Verification items for the finished model (mm, model axes). Face numbers are marked on the shaded views. A direction names the side the tool comes from. Round coordinates to 2 decimals unless told otherwise and drop trailing zeros. Write each loop counter-clockwise with the first axis right and the second up, starting at its lowest first coordinate (ties: lowest second). Pieces come first, ordered by that corner, then holes. Notation, with made-up numbers: (-13, 16) - (13, 16) arc R18 cw to (13, 44) - close; hole circle Ø11 at (30.5, -12.75). An arc over 180 degrees is marked (long way). Answer as a JSON object with one key per item and string values.
```python
from build123d import *

# Parameters (mm, degrees)
SKETCH4_R               = 1.6
BOSS_EXTRUDE1_DEPTH     = 4.8
SKETCH5_R               = 1.6
SKETCH5_R_2             = 0.8
BOSS_EXTRUDE3_DEPTH     = 2
BOSS_EXTRUDE4_DEPTH     = 1.4
CUT_EXTRUDE1_DEPTH      = 1.4
CUT_EXTRUDE1_DEPTH_BACK = 4.6
CHAMFER1_SIZE           = 2.5
FILLET1_R               = 1
CUT_EXTRUDE2_DEPTH      = 10


with BuildPart() as part:
    # Sketch4 → Boss-Extrude1 (new body)
    with BuildSketch(Plane.XY):
        Polygon((183.415148292, 173.842793615), (168.415148292, 173.842793615), (168.415148292, 190.842793615), (183.415148292, 190.842793615), (188.415148292, 190.842793615), (188.415148292, 173.842793615), align=None)
        with Locations((175.415148292, 182.342793615)):
            Circle(SKETCH4_R, mode=Mode.SUBTRACT)
        with Locations((183.415148292, 182.342793615)):
            Circle(SKETCH4_R, mode=Mode.SUBTRACT)
    extrude(amount=BOSS_EXTRUDE1_DEPTH)

    # Sketch5 → Boss-Extrude3 (add)
    with BuildSketch(Plane.XY.offset(4.8)):
        with BuildLine():
            ThreePointArc((158.415148292, 190.842793615), (152.401270103, 182.342793615), (158.415148292, 173.842793615))
            Line((158.415148292, 173.842793615), (188.415148292, 173.842793615))
            Line((188.415148292, 173.842793615), (188.415148292, 190.842793615))
            Line((188.415148292, 190.842793615), (158.415148292, 190.842793615))
        make_face()
        with Locations((175.415148292, 182.342793615)):
            Circle(SKETCH5_R, mode=Mode.SUBTRACT)
        with Locations((183.415148292, 182.342793615)):
            Circle(SKETCH5_R, mode=Mode.SUBTRACT)
        with Locations((161.415148292, 176.342793615)):
            Circle(SKETCH5_R_2, mode=Mode.SUBTRACT)
        with Locations((161.415148292, 188.342793615)):
            Circle(SKETCH5_R_2, mode=Mode.SUBTRACT)
    extrude(amount=BOSS_EXTRUDE3_DEPTH)

    # Sketch6 → Boss-Extrude4 (add)
    with BuildSketch(Plane(origin=(0, 0, 0), x_dir=(-1, 0, 0), z_dir=(0, 0, -1))):
        Polygon((-183.415148292, 189.608806881), (-168.415148292, 189.02555036), (-168.415148292, 190.842793615), (-183.415148292, 190.842793615), (-188.415148292, 190.842793615), (-188.415148292, 189.803225722), align=None)
    extrude(amount=BOSS_EXTRUDE4_DEPTH)

    # Sketch8 → Cut-Extrude1 (cut, two sides: drawn at the far end of the back side and taken through both)
    with BuildSketch(Plane(origin=(0, 0, 0), x_dir=(-1, 0, 0), z_dir=(0, 0, -1)).offset(-CUT_EXTRUDE1_DEPTH_BACK)):
        Polygon((-180.415148292, 190.842793615), (-168.415148292, 177.842793615), (-168.415148292, 190.842793615), align=None)
    extrude(amount=CUT_EXTRUDE1_DEPTH + CUT_EXTRUDE1_DEPTH_BACK, mode=Mode.SUBTRACT)

    # Chamfer1
    # the kernel refuses this chamfer: 2.5 mm, written as the material it takes off along each edge
    with BuildSketch(Plane(origin=(175.415148292, 182.342793615, 6.8), x_dir=(1, 0, 0), z_dir=(0, -1, 0))) as chamfer1_piece_1:
        Polygon((1.6 + CHAMFER1_SIZE, 0), (1.6, -CHAMFER1_SIZE), (1.6, 0), align=None)
    revolve(axis=Axis((175.415148292, 182.342793615, 6.8), (0, 0, 1)), mode=Mode.SUBTRACT)
    with BuildSketch(Plane(origin=(183.415148292, 182.342793615, 6.8), x_dir=(1, 0, 0), z_dir=(0, -1, 0))) as chamfer1_piece_2:
        Polygon((1.6 + CHAMFER1_SIZE, 0), (1.6, -CHAMFER1_SIZE), (1.6, 0), align=None)
    revolve(axis=Axis((183.415148292, 182.342793615, 6.8), (0, 0, 1)), mode=Mode.SUBTRACT)

    # Fillet1
    fillet1_edges = [part.edges().sort_by_distance(p)[0] for p in [
        (168.415148292, 173.842793615, 2.4),
        (188.415148292, 190.842793615, 2.7),
        (188.415148292, 173.842793615, 3.4),
        (158.415148292, 190.842793615, 5.8),
        (158.415148292, 173.842793615, 5.8),
        (180.415148292, 190.842793615, 1.6),
    ]]
    fillet(fillet1_edges, radius=FILLET1_R)

    # Sketch9 → Cut-Extrude2 (cut)
    with BuildSketch(Plane.XY.offset(6.8)):
        Polygon((165.915148292, 186.592793615), (171.915148292, 186.592793615), (171.915148292, 178.092793615), (165.915148292, 178.092793615), (156.915148292, 178.092793615), (156.915148292, 186.592793615), align=None)
    extrude(amount=-CUT_EXTRUDE2_DEPTH, mode=Mode.SUBTRACT)


solid = part.part
```
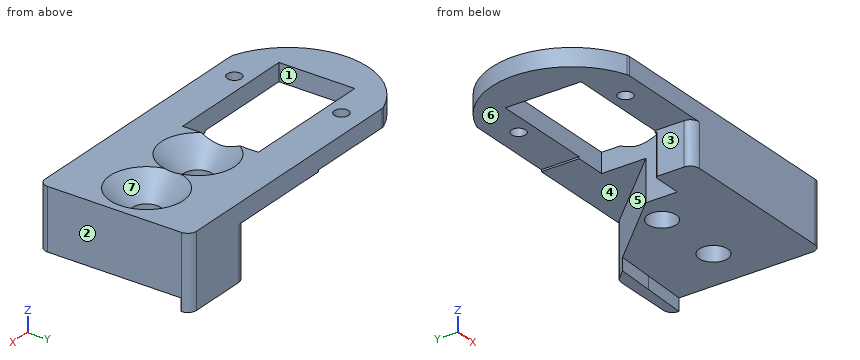
1. Material ranges on probe 1 along Y at (x, z) = (171, 5.25); probe 2 along X at (y, z) = (182, 6.5); probe 3 along X at (y, z) = (185, 6), recorded low to high. Write a range as from..to.
Completed:
{"probe 1": "y = 173.84..178.09, 186.59..190.84", "probe 2": "x = 152.41..156.92, 179.2..179.63, 187.2..188.42", "probe 3": "x = 152.8..156.92, 171.92..173.46, 177.37..181.46, 185.37..188.42"}
2. Cross-section at B-B (z = 3). Record the boundary of the cut face in (x, y), plus the area to 3 significant figures.
Completed:
{"outline": "(168.42, 174.84) arc R1 ccw to (169.42, 173.84) - (187.42, 173.84) arc R1 ccw to (188.42, 174.84) - (188.42, 189.84) arc R1 ccw to (187.42, 190.84) - (180.85, 190.84) arc R1 ccw to (180.12, 190.52) - (171.92, 181.63) - (171.92, 178.09) - (168.65, 178.09) - (168.42, 177.84) - close; hole circle Ø3.2 at (175.42, 182.34); hole circle Ø3.2 at (183.42, 182.34)", "area": "239 mm^2"}
3. Mould release check, pull along X, two halves, no side actions. Record for the marked faces 5, 6 and 7: released by +X, released by -X, zero draft, split by the parting line, or undercut.
Completed:
{"face 5": "released by -X", "face 6": "zero draft", "face 7": "undercut"}
4. Cross-section at A-A (x = 165). Record the boundary of the cut face in (y, z), plus the area to 3 significant figures.
Completed:
{"outline": "(173.84, 4.8) - (178.09, 4.8) - (178.09, 6.8) - (173.84, 6.8) - close; (186.59, 4.8) - (190.84, 4.8) - (190.84, 6.8) - (186.59, 6.8) - close", "area": "17.0 mm^2"}
5. Go/stop test with flat-tipped pins: pin 1 (3.5 mm diameter, centred on x = 175.42, y = 182.34, fed in from -Z); pin 2 (3.5 mm diameter, centred on y = 176.5, z = 3.5, fed in from -X); pin 3 (4 mm diameter, centred on x = 183.42, y = 182.34, fed in from +Z). Record where each tip stops, or that it passes through.
Completed:
{"pin 1": "stops at z = 0", "pin 2": "stops at x = 153.71", "pin 3": "stops at z = 4.71"}
6. Cross-section at C-C (z = 6). Record the boundary of the cut face in (x, y), plus the area to 3 significant figures.
Completed:
{"outline": "(158.24, 173.91) arc R1 ccw to (158.59, 173.84) - (187.42, 173.84) arc R1 ccw to (188.42, 174.84) - (188.42, 189.84) arc R1 ccw to (187.42, 190.84) - (158.59, 190.84) arc R1 ccw to (158.24, 190.78) arc R9.01 ccw to start; hole (156.92, 178.09) - (171.92, 178.09) - (171.92, 186.59) - (156.92, 186.59) - close; hole circle Ø1.6 at (161.42, 176.34); hole circle Ø1.6 at (161.42, 188.34); hole circle Ø6.6 at (175.42, 182.34); hole circle Ø6.6 at (183.42, 182.34)", "area": "384 mm^2"}
7. Access from +Z, -Z, +X, -X, +Y, -Y to the whole of each face (thin tool, end or side, straight path). Record for the marked faces 1, 2, 3 and 4.
Completed:
{"face 1": "+Z, -Z", "face 2": "+Z, -Z, +X, +Y, -Y", "face 3": "-Z, -X, +Y, -Y", "face 4": "-Z, -X, +Y"}
8. Cross-section at D-D (x = 156.5). Record the boundary of the cut face in (y, z).
Completed:
{"outline": "(174.79, 4.8) - (189.9, 4.8) - (189.9, 6.8) - (174.79, 6.8) - close"}
